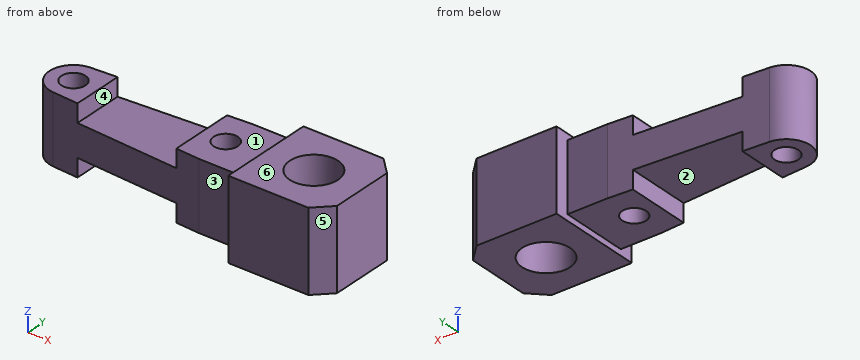
from build123d import *

# Parameters (mm, degrees)
ESQUISSE1_R             = 6
ESQUISSE1_R_2           = 3
BOSS_EXTRU_1_DEPTH      = 20
ESQUISSE3_W             = 16
ESQUISSE3_H             = 17
ESQUISSE3_W_2           = 24.161002882
ESQUISSE3_H_2           = 23.937604634
ENL_V_MAT_EXTRU_1_DEPTH = 1.5
ESQUISSE4_W             = 26
ESQUISSE4_H             = 16.214580426
ENL_V_MAT_EXTRU_2_DEPTH = 6


with BuildPart() as part:
    # Esquisse1 → Boss.-Extru.1 (new body)
    with BuildSketch(Plane.XY):
        Polygon((8, 12), (-12, 12), (-12, -12), (8, -12), (12, -8), (12, 8), align=None)
        Circle(ESQUISSE1_R, mode=Mode.SUBTRACT)
        with BuildLine():
            Line((-12, 8.5), (-22, 8.5))
            Line((-22, 8.5), (-60.391871312, 5.987189397))
            ThreePointArc((-60.391871312, 5.987189397), (-66, 0), (-60.391871312, -5.987189397))
            Line((-60.391871312, -5.987189397), (-22, -8.5))
            Line((-22, -8.5), (-12, -8.5))
            Line((-12, -8.5), (-12, 8.5))
        make_face()
        with Locations((-22, 0)):
            Circle(ESQUISSE1_R_2, mode=Mode.SUBTRACT)
        with Locations((-60, 0)):
            Circle(ESQUISSE1_R_2, mode=Mode.SUBTRACT)
    extrude(amount=BOSS_EXTRU_1_DEPTH)

    # Esquisse3 → Enlèv. mat.-Extru.1 (cut)
    with BuildSketch(Plane.XY.offset(20)):
        with Locations((-20, 0)):
            Rectangle(ESQUISSE3_W, ESQUISSE3_H)
        with Locations((-66.080501441, -0.730031796)):
            Rectangle(ESQUISSE3_W_2, ESQUISSE3_H_2)
    enl_v_mat_extru_1 = extrude(amount=-ENL_V_MAT_EXTRU_1_DEPTH, mode=Mode.SUBTRACT)

    # Esquisse4 → Enlèv. mat.-Extru.2 (cut)
    with BuildSketch(Plane.XY.offset(20)):
        with Locations((-41, 0)):
            Rectangle(ESQUISSE4_W, ESQUISSE4_H)
    enl_v_mat_extru_2 = extrude(amount=-ENL_V_MAT_EXTRU_2_DEPTH, mode=Mode.SUBTRACT)

    # Symétrie1: Enlèv. mat.-Extru.1, Enlèv. mat.-Extru.2 across plane
    add(enl_v_mat_extru_1.mirror(Plane.XY.offset(10)), mode=Mode.SUBTRACT)
    add(enl_v_mat_extru_2.mirror(Plane.XY.offset(10)), mode=Mode.SUBTRACT)


solid = part.part
The model under review builds one solid part; all positions refer to its coordinate system, in mm. Face numbers are marked on the shaded views. A direction names the side the tool comes from. Round coordinates to 2 decimals unless told otherwise and drop trailing zeros. Order: outer loops, then holes, each group sorted by start corner. A loop starts at its lowest first (then second) coordinate and runs counter-clockwise, first axis right, second up. Notation, with made-up numbers: (61.25, 33) -> (76.25, 33) arc R10 cw to (76.25, 49) -> close; hole circle Ø8 at (57.25, 54). An arc over 180 degrees is marked (long way). Write item = value, one per line. Start each with the question number.
Item 1: Consider section A-A on y = 0. Write out the cut boundary in (x, z), plus the area to 3 significant figures.
Item 2: Consider section C-C on z = 9.5. Write out the cut boundary in (x, y).
Item 3: Mouldability with a two-part tool opening along X and no side actions: class the marked faces 4, 5 and 6 as released by +X, released by -X, zero draft, split by the parting line, or undercut.
Item 4: Consider section B-B on x = 0. Write out the cut boundary in (y, z).
Item 5: For the marked faces 1, 2 and 3, list the 3-axis set-ups (+Z, -Z, +X, -X, +Y, -Y) from which the entire face can be reached by the end or side of a thin tool; tool diameter is ignored.
Item 6: For line 1 along Y through (x, z) = (-22, 13); line 2 along X through (y, z) = (2, 13.25); line 3 along X through (y, z) = (-1.75, 9), list the stretches that pass through material, from the lowest coordinate up.
Item 7: Consider section D-D on y = -4.5. Write out the cut boundary in (x, z).
Item 8: Clearance check with flat-ended pins moving along their axes: pin 1 Ø5 at (x, y) = (-44, -0.5) entering from +Z; pin 2 Ø8 at (x, z) = (-17, 6) entering from +Y; pin 3 Ø6 at (x, y) = (-61.5, -2) entering from +Z. State where each tip first meets the part, or that it passes through.
Conclusion:
q1.outline = (-66, 1.5) -> (-63, 1.5) -> (-63, 18.5) -> (-66, 18.5) -> close; (-57, 1.5) -> (-54, 1.5) -> (-54, 6) -> (-28, 6) -> (-28, 1.5) -> (-25, 1.5) -> (-25, 18.5) -> (-28, 18.5) -> (-28, 14) -> (-54, 14) -> (-54, 18.5) -> (-57, 18.5) -> close; (-19, 1.5) -> (-12, 1.5) -> (-12, 0) -> (-6, 0) -> (-6, 20) -> (-12, 20) -> (-12, 18.5) -> (-19, 18.5) -> close; (6, 0) -> (12, 0) -> (12, 20) -> (6, 20) -> close
q1.area = 720 mm2
q2.outline = (-60.39, -5.99) -> (-22, -8.5) -> (-12, -8.5) -> (-12, -12) -> (8, -12) -> (12, -8) -> (12, 8) -> (8, 12) -> (-12, 12) -> (-12, 8.5) -> (-22, 8.5) -> (-60.39, 5.99) arc R6 ccw to start; hole circle Ø6 at (-60, 0); hole circle Ø6 at (-22, 0); hole circle Ø12 at (0, 0)
q3.face_4 = undercut
q3.face_5 = released by +X
q3.face_6 = zero draft
q4.outline = (-12, 0) -> (-6, 0) -> (-6, 20) -> (-12, 20) -> close; (6, 0) -> (12, 0) -> (12, 20) -> (6, 20) -> close
q5.face_1 = +Z, -X, +Y, -Y
q5.face_2 = -Z, +Y, -Y
q5.face_3 = +Z, -Z, -X, -Y
q6.line_1 = -8.5 to -3, 3 to 8.5
q6.line_2 = -65.66 to -62.24, -57.76 to -24.24, -19.76 to -5.66, 5.66 to 12
q6.line_3 = -65.74 to -62.44, -57.56 to -24.44, -19.56 to -5.74, 5.74 to 12
q7.outline = (-63.97, 1.5) -> (-54, 1.5) -> (-54, 6) -> (-28, 6) -> (-28, 1.5) -> (-12, 1.5) -> (-12, 0) -> (-3.97, 0) -> (-3.97, 20) -> (-12, 20) -> (-12, 18.5) -> (-28, 18.5) -> (-28, 14) -> (-54, 14) -> (-54, 18.5) -> (-63.97, 18.5) -> close; (3.97, 0) -> (12, 0) -> (12, 20) -> (3.97, 20) -> close
q8.pin_1 = 14
q8.pin_2 = 8.5
q8.pin_3 = 18.5
